Model file for the job. Use its own axes, mm. A direction names the side the tool comes from. Give positions to 0.01 mm unless a question says otherwise; leave off trailing zeros. Loops run counter-clockwise (first coordinate to the right, second up) from the corner with the lowest first, then second, coordinate; pieces in that order, holes last. Notation, with made-up numbers: M 63.25,0 L 105.25,0 A15 ccw 105.25,18 Z; hole C 46,63 d8. An arc over 180 degrees is marked long. Answer in a Markdown table with one row per item.
```python
from build123d import *

# Parameters (mm, degrees)
SKETCH1_W                = 30
SKETCH1_H                = 5
BOSS_EXTRUDE1_DEPTH      = 35
FILLET1_R                = 15
FILLET3_R                = 5
SKETCH4_R                = 1.5
CUT_EXTRUDE1_DEPTH       = 35
SKETCH5_W                = 6
SKETCH5_H                = 5
SKETCH5_W_2              = 4
SKETCH5_H_2              = 3
BOSS_EXTRUDE2_DEPTH      = 5
CUT_EXTRUDE2_DEPTH       = 5
SKETCH7_R                = 1.5
CUT_EXTRUDE3_DEPTH       = 15
FILLET4_R                = 2.5
BOSS_EXTRUDE3_DEPTH      = 8
BOSS_EXTRUDE3_DEPTH_BACK = 4
SKETCH8_W                = 6
SKETCH8_H                = 4
SKETCH8_W_2              = 5
SKETCH8_H_2              = 3
SKETCH9_W                = 5
SKETCH9_H                = 4.517478875
CUT_EXTRUDE4_DEPTH       = 6
SKETCH10_R               = 1.5
CUT_EXTRUDE5_DEPTH       = 36
FILLET5_R                = 2
FILLET6_R                = 2


with BuildPart() as part:
    # Sketch1 → Boss-Extrude1 (new body)
    with BuildSketch(Plane(origin=(0, 0, 0), x_dir=(1, 0, 0), z_dir=(0, 1, 0))):
        Rectangle(SKETCH1_W, SKETCH1_H)
    extrude(amount=BOSS_EXTRUDE1_DEPTH)

    # Fillet1
    fillet1_edges = [part.edges().sort_by_distance(p)[0] for p in [
        (15, 0, 0),
        (-15, 0, 0),
    ]]
    fillet(fillet1_edges, radius=FILLET1_R - 0.0001)  # a hair under: the kernel refuses the full size

    # Fillet3
    fillet3_edges = [part.edges().sort_by_distance(p)[0] for p in [
        (15, 35, 0),
        (-15, 35, 0),
    ]]
    fillet(fillet3_edges, radius=FILLET3_R)

    # Sketch4 → Cut-Extrude1 (cut)
    with BuildSketch(Plane.ZY.offset(15)):
        with Locations((0, 32)):
            Circle(SKETCH4_R)
    extrude(amount=-CUT_EXTRUDE1_DEPTH, mode=Mode.SUBTRACT)

    # Sketch5 → Boss-Extrude2 (add)
    with BuildSketch(Plane(origin=(0, 35, 0), x_dir=(1, 0, 0), z_dir=(0, 1, 0))):
        Rectangle(SKETCH5_W, SKETCH5_H)
        Rectangle(SKETCH5_W_2, SKETCH5_H_2, mode=Mode.SUBTRACT)
    extrude(amount=BOSS_EXTRUDE2_DEPTH)

    # Sketch6 → Cut-Extrude2 (cut)
    with BuildSketch(Plane(origin=(0, 40, 0), x_dir=(1, 0, 0), z_dir=(0, 1, 0))):
        Polygon((-2, 1.5), (-2, 3.860545562), (2, 3.860545562), (2, -3.417925007), (-2, -3.417925007), align=None)
    extrude(amount=-CUT_EXTRUDE2_DEPTH, mode=Mode.SUBTRACT)

    # Sketch7 → Cut-Extrude3 (cut)
    with BuildSketch(Plane.ZY.offset(3)):
        with Locations((0, 38)):
            Circle(SKETCH7_R)
    extrude(amount=-CUT_EXTRUDE3_DEPTH, mode=Mode.SUBTRACT)

    # Fillet4
    fillet4_edges = [part.edges().sort_by_distance(p)[0] for p in [
        (-2.5, 40, 2.5),
        (-2.5, 40, -2.5),
        (2.5, 40, 2.5),
        (2.5, 40, -2.5),
    ]]
    fillet(fillet4_edges, radius=FILLET4_R - 0.0001)  # a hair under: the kernel refuses the full size

    # Sketch8 → Boss-Extrude3 (add, two sides: drawn at the far end of the back side and taken through both)
    # profile 1 of 2: a face of its own
    with BuildSketch(Plane(origin=(0, 0, 0), x_dir=(1, 0, 0), z_dir=(0, 1, 0)).offset(-BOSS_EXTRUDE3_DEPTH_BACK)):
        with Locations((-10, 0.087771821)):
            Rectangle(SKETCH8_W, SKETCH8_H)
        with Locations((-10, 0.087771821)):
            Rectangle(SKETCH8_W_2, SKETCH8_H_2, mode=Mode.SUBTRACT)
    # profile 2 of 2: a face of its own
    with BuildSketch(Plane(origin=(0, 0, 0), x_dir=(1, 0, 0), z_dir=(0, 1, 0)).offset(-BOSS_EXTRUDE3_DEPTH_BACK)):
        with Locations((10, 0.087771821)):
            Rectangle(SKETCH8_W, SKETCH8_H)
        with Locations((10, 0.087771821)):
            Rectangle(SKETCH8_W_2, SKETCH8_H_2, mode=Mode.SUBTRACT)
    extrude(amount=BOSS_EXTRUDE3_DEPTH + BOSS_EXTRUDE3_DEPTH_BACK)

    # Sketch9 → Cut-Extrude4 (cut)
    with BuildSketch(Plane.XZ.offset(4)):
        with Locations((-10, -0.111234663)):
            Rectangle(SKETCH9_W, SKETCH9_H)
        with Locations((10, -0.111234663)):
            Rectangle(SKETCH9_W, SKETCH9_H)
    extrude(amount=-CUT_EXTRUDE4_DEPTH, mode=Mode.SUBTRACT)

    # Sketch10 → Cut-Extrude5 (cut)
    with BuildSketch(Plane.ZY.offset(13)):
        with Locations(Location((-0.087771821, -2, 0), (0, 0, 180))):
            Circle(SKETCH10_R)
    extrude(amount=-CUT_EXTRUDE5_DEPTH, mode=Mode.SUBTRACT)

    # Fillet5
    fillet5_edges = [part.edges().sort_by_distance(p)[0] for p in [
        (7.25, -4, -2.087771821),
        (7.25, -4, 1.912228179),
        (12.75, -4, 1.912228179),
        (12.75, -4, -2.087771821),
    ]]
    fillet(fillet5_edges, radius=FILLET5_R - 0.0001)  # a hair under: the kernel refuses the full size

    # Fillet6
    fillet6_edges = [part.edges().sort_by_distance(p)[0] for p in [
        (-7.25, -4, 1.912228179),
        (-12.75, -4, 1.912228179),
        (-12.75, -4, -2.087771821),
        (-7.25, -4, -2.087771821),
    ]]
    fillet(fillet6_edges, radius=FILLET6_R - 0.0001)  # a hair under: the kernel refuses the full size


solid = part.part
```
(1) Saw through at A-A, the plane y = 38. Give the cut face in (x, z).
Established:
| item | result |
|---|---|
| outline | M -3,-2.45 L -2,-2.45 L -2,-1.5 L -3,-1.5 Z; M -3,1.5 L -2,1.5 L -2,2.45 L -3,2.45 Z; M 2,-2.45 L 3,-2.45 L 3,-1.5 L 2,-1.5 Z; M 2,1.5 L 3,1.5 L 3,2.45 L 2,2.45 Z |
(2) Which spindle directions (+Z, -Z, +X, -X, +Y, -Y) get a long thin tool onto all of the face, cutting with end or side? Do faces 1 (the flat face through (10.9, 2.4, 1.912)), 2 (the flat face through (11, 3, -1.588)), 3 (the flat face through (2, 36, 0)), 4 (the flat face through (-11, 3, -2.088)). Say none if no direction does.
Established:
| item | result |
|---|---|
| face 1 | +Z, +X, -Y |
| face 2 | -Y |
| face 3 | +Z, -Z, +Y |
| face 4 | -Z, -X, -Y |
(3) Mould opens along Y. For faces 5 (the flat face through (7.5, 0, 0)), 6 (the cylindrical face through (12.754, -3.399, -1.517)), 7 (the cylindrical face through (-2.507, 36.536, -0.325)) say: pulls with the +Y half, pulls with the -Y half, needs draft (parallel to the pull), parting line crosses it, or undercut.
Established:
| item | result |
|---|---|
| face 5 | needs draft |
| face 6 | pulls with the -Y half |
| face 7 | undercut |
(4) Saw through at D-D, the plane z = 0.65. Count the separate pieces of the cut face and the enclosed holes in it, and give its area (3 significant figures).
Established:
| item | result |
|---|---|
| separate pieces | 8 |
| enclosed holes | 0 |
| area | 880 mm2 |
(5) Saw through at C-C, the plane x = -9.5. Give the cut face in (y, z), and give its area (3 significant figures).
Established:
| item | result |
|---|---|
| outline | M 2,-2.09 L 3.39,-2.09 L 3.39,-2.5 L 35,-2.5 L 35,2.5 L 3.39,2.5 L 3.39,1.91 L 2,1.91 L 2,1.41 L 3.39,1.41 L 3.39,-1.59 L 2,-1.59 Z; hole C 32,0 d3 |
| area | 152 mm2 |
(6) Flat gauge pins, fed straight in: P1, Ø5, axis at x = -8.5, y = 2, coming from the -Z side; P2, Ø1, axis at y = 6.5, z = -1, coming from the -X side; P3, Ø2.5, axis at x = 5, z = 0, coming from the +Y side; P4, Ø2.5, axis at y = 37, z = -0.5, coming from the +X side. Where does each tip first touch, or does it go through?
Established:
| item | result |
|---|---|
| P1 | stops at z = -2.5 |
| P2 | stops at x = -13 |
| P3 | stops at y = 35 |
| P4 | stops at x = 3 |
(7) Saw through at B-B, the plane y = 32. Give the cut face in (x, z), and give its area (3 significant figures).
Established:
| item | result |
|---|---|
| outline | M -14.58,-2.5 L 14.58,-2.5 L 14.58,-1.5 L -14.58,-1.5 Z; M -14.58,1.5 L 14.58,1.5 L 14.58,2.5 L -14.58,2.5 Z |
| area | 58.3 mm2 |
(8) Wall check: L1, parallel to Y at x = -0.5, z = 0; L2, parallel to Y at x = -7, z = 1.95; L3, parallel to Y at x = 1, z = 1.15. Give the ranges that are in metal, low to high.
Established:
| item | result |
|---|---|
| L1 | y = 0.01 to 30.5, 33.5 to 35 |
| L2 | y = 1.73 to 35 |
| L3 | y = 0.03 to 31.04, 32.96 to 35 |
